from build123d import *

# Parameters (mm, degrees)
EXTRUDE_1_DEPTH     = 3
CUT_EXTRUDE_START   = -5
CUT_EXTRUDE_1_DEPTH = 1.95


with BuildPart() as part:
    # 草圖1 → 填料-伸長1 (new body)
    with BuildSketch(Plane(origin=(0, 0, 0), x_dir=(1, 0, 0), z_dir=(0, 1, 0))):
        Polygon((22, 5.315789474), (22, 20.315789474), (62, 20.315789474), (62, -19.684210526), (22, -19.684210526), (22, -4.684210526), (-28, -4.684210526), (-28, 5.315789474), align=None)
    extrude(amount=EXTRUDE_1_DEPTH)

    # 草圖3 → 除料-伸長1 (cut, symmetric)
    with BuildSketch(Plane.XY.offset(4.684210526).offset(CUT_EXTRUDE_START)):
        Polygon((-15.649759089, 3), (-1.192153505, 3), (-0.217394417, 0), (-14.675, 0), align=None)
    extrude(amount=CUT_EXTRUDE_1_DEPTH, both=True, mode=Mode.SUBTRACT)


solid = part.part
Could you check a few things on this model? Use its own coordinates, in mm. A direction names the side the tool comes from. Give positions to 0.01 mm unless a question says otherwise; leave off trailing zeros. Loops run counter-clockwise (first coordinate to the right, second up) from the corner with the lowest first, then second, coordinate; pieces in that order, holes last. Notation, with made-up numbers: (-14.75, 50.25) -> (7.25, 50.25) arc R32 ccw to (7.25, 78.25) -> close; hole circle Ø1 at (82, 28.5). An arc over 180 degrees is marked (long way). Return JSON: item names as keys, results as strings.
Item 1: We'd pull the mould along X, two halves only. Please class faces 1 (the flat face through (28, 0, -1)), 2 (the flat face through (-15, 1, 0)), 3 (the flat face through (-0.71, 1.52, -0.29)), 4 (the flat face through (-28, 1, 0)): +X half, -X half, draft (parallel to the pull), parting line (faces both ways), or undercut.
Geometry results:
{"face 1": "draft", "face 2": "undercut", "face 3": "undercut", "face 4": "-X half"}
Item 2: If we section it at D-D on x = 17: List the corners of the cut face in (y, z) for me.
Geometry results:
{"outline": "(0, -5.32) -> (3, -5.32) -> (3, 4.68) -> (0, 4.68) -> close"}
Item 3: If we section it at A-A on x = -7: List the corners of the cut face in (y, z) for me.
Geometry results:
{"outline": "(0, -5.32) -> (3, -5.32) -> (3, -2.27) -> (0, -2.27) -> close; (0, 1.63) -> (3, 1.63) -> (3, 4.68) -> (0, 4.68) -> close"}
Item 4: If we section it at B-B on z = -17: List the corners of the cut face in (x, y) for me.
Geometry results:
{"outline": "(22, 0) -> (62, 0) -> (62, 3) -> (22, 3) -> close"}
Item 5: I'm going to push flat-ended pins straight in: pin 1 (1.5 mm diameter, centred on x = -4.5, y = 2, fed in from -Z); pin 2 (0.9 mm diameter, centred on x = -8.5, y = 2, fed in from +Z). Where does each tip first touch, or does it pass through?
Geometry results:
{"pin 1": "stops at z = -5.32", "pin 2": "stops at z = 4.68"}
Item 6: Which directions (+Z, -Z, +X, -X, +Y, -Y) give clear straight access to the entire face, cutting with the end or side of a thin tool? Please do faces 5 (the flat face through (62, 1, -1)), 6 (the flat face through (22, 1, 12)), 7 (the flat face through (22, 1, -13)).
Geometry results:
{"face 5": "+Z, -Z, +X, +Y, -Y", "face 6": "+Z, -X, +Y, -Y", "face 7": "-Z, -X, +Y, -Y"}
Item 7: If we section it at C-C on y = 2.55: List the corners of the cut face in (x, z) for me.
Geometry results:
{"outline": "(-28, -5.32) -> (22, -5.32) -> (22, -20.32) -> (62, -20.32) -> (62, 19.68) -> (22, 19.68) -> (22, 4.68) -> (-28, 4.68) -> close; hole (-15.5, -2.27) -> (-1.05, -2.27) -> (-1.05, 1.63) -> (-15.5, 1.63) -> close"}
Item 8: I need wall thicknesses on L1, parallel to Z at x = -7.5, y = 2.2; L2, parallel to X at y = 0.25, z = 15.5; L3, parallel to Z at x = 13, y = 0.65. Which ranges of each line are inside material? Lowest first, please. Write a range as from..to.
Geometry results:
{"L1": "z = -5.32..-2.27, 1.63..4.68", "L2": "x = 22..62", "L3": "z = -5.32..4.68"}
